Design review of the part built by this model. Coordinates are the model's own, in mm. Face numbers are marked on the shaded views. A direction names the side the tool comes from. Coordinates: 2 decimals unless noted, no trailing zeros. Loops run counter-clockwise (first coordinate to the right, second up) from the corner with the lowest first, then second, coordinate; pieces in that order, holes last. Notation, with made-up numbers: (83, 6) - (133, 6) arc R22 cw to (133, 34) - close; hole circle Ø3 at (77, -8). An arc over 180 degrees is marked (long way). Use one line per item in the form item = value. Start each with the question number.
(1) Add section A-A (y = 2.5). State the section outline as (x, z) points.
(2) Tool access review of the marked faces 4, 5 and 6: name each direction out of +Z, -Z, +X, -X, +Y, -Y from which nothing blocks a thin tool from reaching the whole face with its end or side.
(3) The part is to be moulded in two halves that separate along Y. For the marked faces 1, 2 and 3, say which applies: pulls with the +Y half, pulls with the -Y half, needs draft (parallel to the pull), parting line crosses it, or undercut.
(4) For L1, parallel to Y at x = -5, z = 25; L2, parallel to Y at x = 13.5, z = 28.5; L3, parallel to X at y = 41.5, z = 10.5, list the stretches that pass through material, from the lowest coordinate up.
(5) Add section C-C (z = 9). State the section outline as (x, y) points (3 decimals).
(6) Add section B-B (x = 0). State the section outline as (y, z) points, plus the area to 3 significant figures.
(7) Clearance check with flat-ended pins moving along their axes: pin 1 Ø1.3 at (y, z) = (45.5, 20) entering from +X; pin 2 Ø12 at (x, z) = (10, 10) entering from +Y; pin 3 Ø2 at (y, z) = (42.5, 9) entering from +X. State where each tip first meets the part, or that it passes through.
(8) Add section D-D (y = 47). State the section outline as (x, z) points, plus the area to 3 significant figures.
Autodesk Fusion 360 part; units mm, degrees
sketch "Sketch1" plane through (0, 0, 0) normal (0, 1, 0) x (1, 0, 0)
  line L0 (0, 0) -> (44, 0)
  line L1 (44, 0) -> (44, -35)
  line L2 (44, -35) -> (0, -35)
  line L3 (0, -35) -> (0, 0)
  line L4 (0, 0) -> (-5, 0)
  line L5 (0, -35) -> (-5, -35)
  line L6 (-5, -35) -> (-5, 0)
  dimension "d1" = 44
  dimension "d2" = 35
  dimension "d3" = 5
  dimension "d4" = 5
extrude "Extrude1" add sketch "Sketch1" along normal blind 49 contours L3 L4 L5 L6 makes body 1
sketch "Sketch2" plane through (0, 0, 0) normal (0, 1, 0) x (1, 0, 0)
  line L0 (0, 0) -> (44, 0)
  line L1 (44, 0) -> (44, -35)
  line L2 (44, -35) -> (0, -35)
  line L3 (0, -35) -> (0, 0)
  dimension "d7" = 44
extrude "Extrude2" add sketch "Sketch2" against normal blind 2 separate body makes body 2
extrude "Extrude3" add 1 faces at (-3.3333, 0, 11.6667) along direction (0, -1, 0) blind 2 on bodies 1 bodies 1 2
extrude "Extrude4" cut 1 faces at (-5, 15, 23.3333) along direction (1, 0, 0) blind 3 on bodies 1 bodies 1
extrude "Extrude5" add 1 faces at (14, -2, 11.6667) along direction (0, -1, 0) blind 3 on bodies 1 bodies 1
extrude "Extrude6" add 1 faces at (-2, 13, 11.6667) along direction (-1, 0, 0) blind 3 on bodies 1 bodies 1
sketch "Sketch3" plane through (0, 0, 0) normal (0, 0, 1) x (1, 0, 0)
  line L0 (40, 0) -> (44, 0)
  line L1 (0, 49) -> (7, 49)
  curve L2
  curve L3
  curve L4
  curve L5
  curve L6
  curve L7
  curve L8
  curve L9
  curve L10
  curve A0
  curve A1
  curve L11
  curve L12
  curve L13
  curve L14
  curve L15
  curve L16
  curve L17
  curve L18
  curve L19
  curve L20
  curve L21
  curve L22
  curve A2
  curve L23
  line L24 (40, 0) -> (0, 0)
  line L25 (0, 0) -> (0, 45)
  line L26 (40, 0) -> (0, 0)
  line L27 (0, 0) -> (0, 45)
  line L28 (44, 0) -> (40, 0)
  line L29 (40, 0) -> (40, 5)
  line L30 (40, 5) -> (44, 5)
  line L31 (44, 5) -> (44, 0)
  line L32 (40, 5) -> (44, 5)
  line L33 (44, 5) -> (44, 7)
  line L34 (44, 7) -> (40, 7)
  line L35 (40, 7) -> (40, 5)
  circle A3 centre (42, 6.165) radius 1.165
  point P0 (44, 0)
  point P1 (44, 0)
  point P2 (0.0061, 44.9497)
  dimension "d77" = 5
  dimension "d78" = 4
  dimension "d79" = 2
  dimension "d80" = 2.33
extrude "Extrude9" add sketch "Sketch3" along normal blind 35 contours L0 L28 L29 L30 L31 L32 | L30 L32 L34 L35 A3 | L30 L32 L33 L34 A3 bodies 1
extrude "Extrude10" cut 1 faces at (0, 16.3333, 23.3333) along direction (-1, 0, 0) blind 1 on bodies 1 bodies 1
extrude "Extrude11" add 1 faces at (-5, 13, 11.6667) along direction (-1, 0, 0) blind 1 on bodies 1 bodies 1
extrude "Extrude13" add 1 faces at (-6, 13, 11.6667) along direction (-1, 0, 0) blind 5 on bodies 1 bodies 1
extrude "Extrude14" cut 1 faces at (-1, 16.3333, 23.3333) along direction (-1, 0, 0) blind 5 on bodies 1 bodies 1
sketch "Sketch5" plane through (0, 0, 0) normal (0, 0, 1) x (1, 0, 0)
  line L0 (1, 49) -> (-1, 49)
  line L1 (1, 45) -> (1, 49)
  line L2 (-1, 45) -> (1, 45)
  circle A0 centre (0.165, 47) radius 1.165
  line L3 (-1, 49) -> (-1, 45)
  line L4 (-6, 49) -> (-1, 49)
  line L5 (-6, 45) -> (-6, 49)
  line L6 (-6, 49) -> (-6, 45)
  line L7 (-1, 45) -> (-6, 45)
  line L8 (-1, 49) -> (-1, 45)
  point P0 (-6, 49)
  point P1 (-6, 45)
  point P2 (-6, 45)
  dimension "d87" = 5
  dimension "d88" = 4
  dimension "d89" = 2
  dimension "d90" = 2.33
extrude "Extrude15" add sketch "Sketch5" along normal blind 35 contours L0 L1 A0 L3 L8 | L3 L4 L5 L6 L7 L8 | L1 L2 A0 L3 L8 bodies 1
extrude "Extrude12" [suppressed]
extrude "Extrude7" [suppressed]
sketch "Sketch4" plane through (0, 0, 0) normal (0, 0, 1) x (1, 0, 0)
  line L0 (7.33, 45) -> (7.33, 49)
  line L1 (9.33, 49) -> (7.33, 49)
  line L2 (0, 49) -> (0, 45)
  line L3 (0, 45) -> (7.33, 45)
  line L4 (7.33, 45) -> (7.33, 49)
  line L5 (9.33, 45) -> (9.33, 49)
  line L6 (0, 45) -> (7.33, 45)
  line L7 (7.33, 49) -> (0, 49)
  line L8 (7.33, 49) -> (7.33, 45)
  circle A0 centre (8.495, 47) radius 1.165
  circle A1 centre (8.495, 47) radius 1.165
  line L9 (9.33, 45) -> (9.33, 49)
  line L10 (7.33, 49) -> (0, 49)
  line L11 (7.33, 49) -> (7.33, 45)
  line L12 (7.33, 45) -> (9.33, 45)
  line L13 (7.33, 45) -> (7.33, 49)
  line L14 (9.33, 49) -> (7.33, 49)
  line L15 (7.33, 45) -> (9.33, 45)
  line L16 (7.33, 45) -> (9.33, 45)
  line L17 (7.33, 49) -> (0, 49)
  line L18 (0, 45) -> (7.33, 45)
  line L19 (7.33, 49) -> (7.33, 45)
  line L20 (9.33, 45) -> (9.33, 49)
  circle A2 centre (8.495, 47) radius 1.165
  line L21 (9.33, 49) -> (7.33, 49)
  point P0 (0, 45)
  dimension "d66" = 7.33
  dimension "d67" = 4
  dimension "d68" = 2
  dimension "d69" = 7.33
  dimension "d70" = 4
  dimension "d71" = 2
  dimension "d72" = 7.33
  dimension "d73" = 4
  dimension "d74" = 2
extrude "Extrude8" [suppressed]
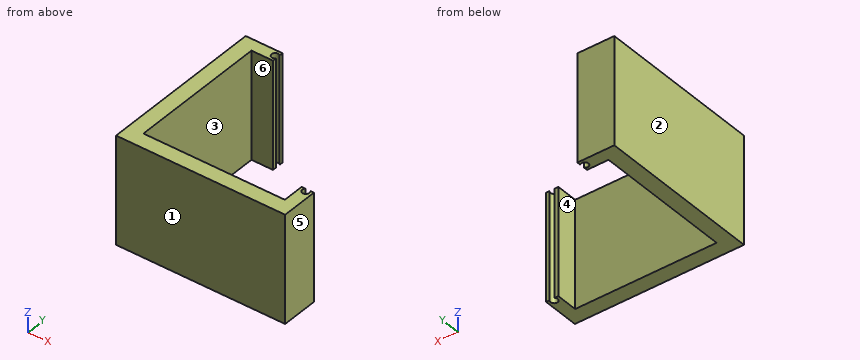
Computed values:
q1.outline = (-11, 0) - (-6, 0) - (-6, 35) - (-11, 35) - close; (40, 0) - (44, 0) - (44, 35) - (40, 35) - close
q2.face_4 = +Z, -Z, +Y
q2.face_5 = +Z, -Z, +X, +Y, -Y
q2.face_6 = +Z, -Z, +X
q3.face_1 = pulls with the -Y half
q3.face_2 = needs draft
q3.face_3 = undercut
q4.L1 = -5 to 0, 45 to 49
q4.L2 = -5 to 0
q4.L3 = -11 to -6
q5.outline = (-11, -5) - (44, -5) - (44, 7) - (42.812, 7) arc R1.165 cw (long way) to (41.188, 7) - (40, 7) - (40, 0) - (-6, 0) - (-6, 45) - (1, 45) - (1, 46.188) arc R1.165 cw (long way) to (1, 47.812) - (1, 49) - (-11, 49) - close
q6.outline = (-5, 0) - (0, 0) - (0, 35) - (-5, 35) - close; (45, 0) - (45.85, 0) - (45.85, 35) - (45, 35) - close; (48.15, 0) - (49, 0) - (49, 35) - (48.15, 35) - close
q6.area = 234 mm^2
q7.pin_1 = 1
q7.pin_2 = 0
q7.pin_3 = -6
q8.outline = (-11, 0) - (-1, 0) - (-1, 35) - (-11, 35) - close
q8.area = 350 mm^2
